Autodesk Inventor part; units mm, degrees
ref_plane "YZ Plane" through (0, 0, 0) normal (1, 0, 0) x (0, 1, 0)
ref_plane "XZ Plane" through (0, 0, 0) normal (0, 1, 0) x (-1, 0, 0)
ref_plane "XY Plane" through (0, 0, 0) normal (0, 0, 1) x (1, 0, 0)
sketch "Эскиз1" plane through (0, 0, 0) normal (0, 1, 0) x (-1, 0, 0)
  line L0 (-110, 90) -> (110, 90)
  line L1 (110, 90) -> (110, -90)
  line L2 (110, -90) -> (-110, -90)
  line L3 (-110, -90) -> (-110, 90)
  line L4 (-110, 90) -> (110, -90) construction
  line L5 (110, 90) -> (-110, -90) construction
  point P0 (0, 0)
  dimension "d0" = 220
  dimension "d1" = 180
extrude "Выдавливание1" add sketch "Эскиз1" along normal blind 3
sketch "Эскиз2" plane through (0, 0, 0) normal (0, -1, 0) x (1, 0, 0)
  circle A0 centre (99.9996, -40) radius 2
  circle A1 centre (99.9996, 0) radius 2
  circle A2 centre (99.9996, 40) radius 2
  circle A3 centre (-99.9997, 0) radius 2
  circle A4 centre (-99.9997, -40) radius 2
  circle A5 centre (-99.9997, 40) radius 2
  point P0 (0, 0)
extrude "Выдавливание2" cut sketch "Эскиз2" against normal blind 3
sketch "Эскиз3" plane through (0, 3, 0) normal (0, 1, 0) x (1, 0, 0)
  circle A0 centre (87.4999, 80.5) radius 2
  circle A1 centre (-87.5001, 80.5) radius 2
  circle A2 centre (-87.5001, -80.5) radius 2
  circle A3 centre (87.4999, -80.5) radius 2
  point P0 (0, 0)
extrude "Выдавливание3" cut sketch "Эскиз3" against normal blind 10
sketch "Эскиз4" plane through (0, 3, 0) normal (0, 1, 0) x (1, 0, 0)
  circle A0 centre (-31.6806, 0) radius 15
  point P0 (0, 0)
extrude "Выдавливание4" cut sketch "Эскиз4" against normal blind 10
properties part number "000.003 - cap"
Source: CAD feature listing. Evaluate the final solid. Frame: model axes, mm. Round coordinates to 2 decimals unless told otherwise and drop trailing zeros. Loops run counter-clockwise (first coordinate to the right, second up) from the corner with the lowest first, then second, coordinate; pieces in that order, holes last.
1. Section query B-B on y = 1.2. Give the number of separate pieces and of enclosed holes in the cut face, and give its area (3 significant figures).
2. Ray query, L1, parallel to X at y = 2.25, z = -80.5; L2, parallel to Z at x = -30.5, y = 0.35; L3, parallel to Z at x = 99, y = 0.7. Return the intervals inside material, ascending.
3. Mould query, pull axis Z, two halves, no side actions, for faces 1 (the flat face through (2, 0, 1)), 2 (the cylindrical face through (-34.932, 1.521, 14.643)). Classes: released by +Z, released by -Z, zero draft, split by the parting line, or undercut.
4. Section query C-C on z = 9.5. Output: boundary loops of the cut face in (x, y), and give its area (3 significant figures).
5. Section query A-A on x = -19.5. Output: boundary loops of the cut face in (y, z), and give its area (3 significant figures).
Answers below:
1. separate pieces: 1
1. enclosed holes: 11
1. area: 38,800 mm2
2. L1: x = -110 to -89.5, -85.5 to 85.5, 89.5 to 110
2. L2: z = -90 to -14.95, 14.95 to 90
2. L3: z = -90 to -41.73, -38.27 to -1.73, 1.73 to 38.27, 41.73 to 90
3. face 1: zero draft
3. face 2: undercut
4. outline: (-110, 0) - (-43.29, 0) - (-43.29, 3) - (-110, 3) - close; (-20.07, 0) - (110, 0) - (110, 3) - (-20.07, 3) - close
4. area: 590 mm2
5. outline: (0, -90) - (3, -90) - (3, -8.75) - (0, -8.75) - close; (0, 8.75) - (3, 8.75) - (3, 90) - (0, 90) - close
5. area: 487 mm2
